```python
from build123d import *

# Parameters (mm, degrees)
SKETCH1_R           = 22.5
BOSS_EXTRUDE1_DEPTH = 20
SKETCH11_W          = 62.5
SKETCH11_H          = 45
BOSS_EXTRUDE4_DEPTH = 10
SKETCH6_R           = 15
BOSS_EXTRUDE2_DEPTH = 10
SKETCH7_R           = 12.5
CUT_EXTRUDE1_DEPTH  = 10
SKETCH8_R           = 2
CUT_EXTRUDE3_DEPTH  = 70.372184628
SKETCH9_R           = 2.5
CUT_EXTRUDE4_DEPTH  = 10
SKETCH12_W          = 16
SKETCH12_H          = 45
BOSS_EXTRUDE5_DEPTH = 70
SKETCH13_W          = 14
SKETCH13_H          = 43
CUT_EXTRUDE5_DEPTH  = 5
SKETCH14_W          = 9
SKETCH14_H          = 9
SKETCH14_W_2        = 14
SKETCH14_H_2        = 16
CUT_EXTRUDE6_DEPTH  = 6
CUT_EXTRUDE7_DEPTH  = 10


with BuildPart() as part:
    # Sketch1 → Boss-Extrude1 (new body)
    with BuildSketch(Plane.XY):
        Circle(SKETCH1_R)
    extrude(amount=BOSS_EXTRUDE1_DEPTH)

    # Sketch11 → Boss-Extrude4 (add)
    with BuildSketch(Plane.XY):
        with Locations((31.25, 0)):
            Rectangle(SKETCH11_W, SKETCH11_H)
    extrude(amount=BOSS_EXTRUDE4_DEPTH)

    # Sketch6 → Boss-Extrude2 (add)
    with BuildSketch(Plane.XY.offset(20)):
        Circle(SKETCH6_R)
    extrude(amount=BOSS_EXTRUDE2_DEPTH)

    # Sketch7 → Cut-Extrude1 (cut)
    with BuildSketch(Plane.XY.offset(30)):
        Circle(SKETCH7_R)
    extrude(amount=-CUT_EXTRUDE1_DEPTH, mode=Mode.SUBTRACT)

    # Sketch8 → Cut-Extrude3 (cut, through all)
    with BuildSketch(Plane.XY.offset(20)):
        with Locations((-10, 0)):
            Circle(SKETCH8_R)
        with Locations(Location((10, 0, 0), (0, 0, 180))):
            Circle(SKETCH8_R)
    extrude(amount=-CUT_EXTRUDE3_DEPTH, mode=Mode.SUBTRACT)

    # Sketch9 → Cut-Extrude4 (cut)
    with BuildSketch(Plane.XY.offset(20)):
        with Locations((0, 18)):
            Circle(SKETCH9_R)
        with Locations((-12.727922061, -12.727922061)):
            Circle(SKETCH9_R)
        with Locations((12.727922061, -12.727922061)):
            Circle(SKETCH9_R)
    extrude(amount=-CUT_EXTRUDE4_DEPTH, mode=Mode.SUBTRACT)

    # Sketch12 → Boss-Extrude5 (add)
    with BuildSketch(Plane.XY.offset(10)):
        with Locations((54.5, 0)):
            Rectangle(SKETCH12_W, SKETCH12_H)
    extrude(amount=BOSS_EXTRUDE5_DEPTH)

    # Sketch13 → Cut-Extrude5 (cut)
    with BuildSketch(Plane.XY.offset(80)):
        with Locations((54.5, -1)):
            Rectangle(SKETCH13_W, SKETCH13_H)
    extrude(amount=-CUT_EXTRUDE5_DEPTH, mode=Mode.SUBTRACT)

    # Sketch14 → Cut-Extrude6 (cut)
    with BuildSketch(Plane.XY.offset(75)):
        with Locations((52, 4)):
            Rectangle(SKETCH14_W, SKETCH14_H)
        with Locations((54.5, -14.5)):
            Rectangle(SKETCH14_W_2, SKETCH14_H_2)
    extrude(amount=-CUT_EXTRUDE6_DEPTH, mode=Mode.SUBTRACT)

    # Sketch17 → Cut-Extrude7 (cut)
    with BuildSketch(Plane(origin=(0, 0, 0), x_dir=(-1, 0, 0), z_dir=(0, 0, -1))):
        Polygon((-10, 2), (-10, 4), (24, 4), (24, -4), (-10, -4), (-10, -2), align=None)
    extrude(amount=-CUT_EXTRUDE7_DEPTH, mode=Mode.SUBTRACT)


solid = part.part
```
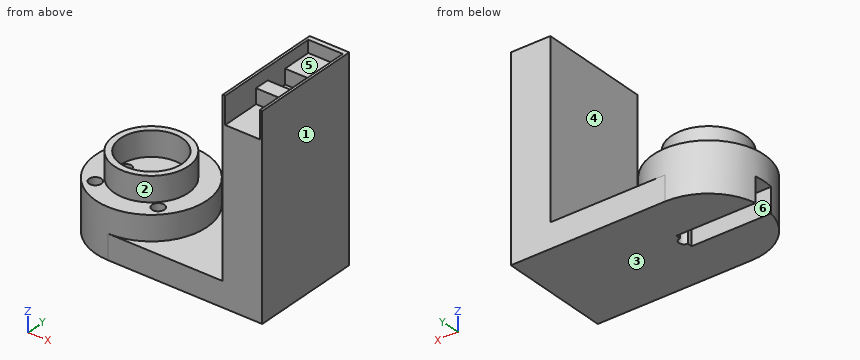
Here's how the part is built. I have some questions about the finished solid (model axes, mm). Face numbers are marked on the shaded views. A direction names the side the tool comes from. Round coordinates to 2 decimals unless told otherwise and drop trailing zeros. Write each loop counter-clockwise with the first axis right and the second up, starting at its lowest first coordinate (ties: lowest second). Pieces come first, ordered by that corner, then holes.
Q1. Which directions (+Z, -Z, +X, -X, +Y, -Y) give clear straight access to the entire face, cutting with the end or side of a thin tool? Please do the marked faces 4, 5 and 6.
Q2. Will these pins go through, and if not, where does the flat tip stop? P1, Ø5.5, axis at x = -13.5, y = -13, coming from the +Z side; P2, Ø4, axis at x = 11, y = 12, coming from the +Z side; P3, Ø5.5, axis at x = 53, z = 78.5, coming from the -Y side.
Q3. If we section it at C-C on z = 32.5: Write out the boundary of the cut face in (x, y).
Q4. If we mould it in two halves opening along X, with no side actions, what happens to the marked faces 1, 2 and 3? For each: +X half, -X half, draft (parallel to the pull), parting line (faces both ways), or undercut.
Q5. If we section it at D-D on y = -18: Write out the boundary of the cut face in (x, z), plus the area to 3 significant figures.
Q6. If we section it at B-B on x = 53: Write out the boundary of the cut face in (y, z).
Q7. If we section it at A-A on y = 18: Write out the boundary of the cut face in (x, z), plus the area to 3 significant figures.
Q8. Please list where these lines run through material, in increasing order: probe 1 along X at (y, z) = (0.5, 21); probe 2 along Y at (x, z) = (0, 17); probe 3 along X at (y, z) = (-11.5, 26.5).
Answer below:
1. face 4: +Z, +Y, -Y
1. face 5: +Z, -Y
1. face 6: -Z, -X
2. P1: stops at z = 20
2. P2: stops at z = 30
2. P3: stops at y = 20.5
3. outline: (46.5, -22.5) - (62.5, -22.5) - (62.5, 22.5) - (46.5, 22.5) - close
4. face 1: +X half
4. face 2: undercut
4. face 3: draft
5. outline: (-13.5, 0) - (62.5, 0) - (62.5, 80) - (61.5, 80) - (61.5, 69) - (47.5, 69) - (47.5, 80) - (46.5, 80) - (46.5, 10) - (13.5, 10) - (13.5, 20) - (-13.5, 20) - close
5. area: 2,000 mm2
6. outline: (-22.5, 0) - (22.5, 0) - (22.5, 80) - (20.5, 80) - (20.5, 75) - (8.5, 75) - (8.5, 69) - (-0.5, 69) - (-0.5, 75) - (-6.5, 75) - (-6.5, 69) - (-22.5, 69) - close
7. outline: (-13.5, 0) - (62.5, 0) - (62.5, 80) - (61.5, 80) - (61.5, 75) - (47.5, 75) - (47.5, 80) - (46.5, 80) - (46.5, 10) - (13.5, 10) - (13.5, 20) - (2.5, 20) - (2.5, 10) - (-2.5, 10) - (-2.5, 20) - (-13.5, 20) - close
7. area: 2,030 mm2
8. probe 1: x = -14.99 to -12.49, 12.49 to 14.99, 46.5 to 62.5
8. probe 2: y = -22.5 to 15.5, 20.5 to 22.5
8. probe 3: x = -9.63 to -4.9, 4.9 to 9.63, 46.5 to 62.5
